Part print with two shaded views. Sizes in mm from the minimum x, y, z corner. A direction names the side the tool comes from. Round coordinates to 2 decimals unless told otherwise and drop trailing zeros. Write each loop counter-clockwise with the first axis right and the second up, starting at its lowest first coordinate (ties: lowest second). Pieces come first, ordered by that corner, then holes. Notation, with made-up numbers: M 51,2 L 58,2 A15 ccw 58,6 Z; hole C 48.25,78 d10. An arc over 180 degrees is marked long. One line per question, with ' | ' between items. Start each with the question number.
1) Mould opens along Y. For the marked faces 5, 6 and 7 say: pulls with the +Y half, pulls with the -Y half, needs draft (parallel to the pull), parting line crosses it, or undercut.
2) Wall check: probe 1 along Y at (x, z) = (84.5, 96.5); probe 2 along X at (y, z) = (21, 50); probe 3 along Z at (x, y) = (85, 14.75). Give the ranges that are in metal, low to high. Write a range as [from, to].
3) Tool access for the marked faces 1, 2, 3 and 4: list every direction of +Z, -Z, +X, -X, +Y, -Y with a clear straight run to the whole face (end or side of a thin tool).
4) Saw through at A-A (z = 80.5). List the corners of the cut face in (x, y).
5) Drop flat-ended pins along their axis: pin 1 Ø1.5 at (x, z) = (93.5, 89) entering from -Y; pin 2 Ø3 at (y, z) = (53, 62.5) entering from +X; pin 3 Ø22 at (y, z) = (22, 64) entering from -X. Give the stop position or say it passes through.
6) Saw through at B-B (x = 85). List the corners of the cut face in (y, z), plus the area to 3 significant figures.
7) Saw through at C-C (y = 56.5). List the corners of the cut face in (x, z).
8) Saw through at D-D (x = 63). List the corners of the cut face in (y, z), plus the area to 3 significant figures.
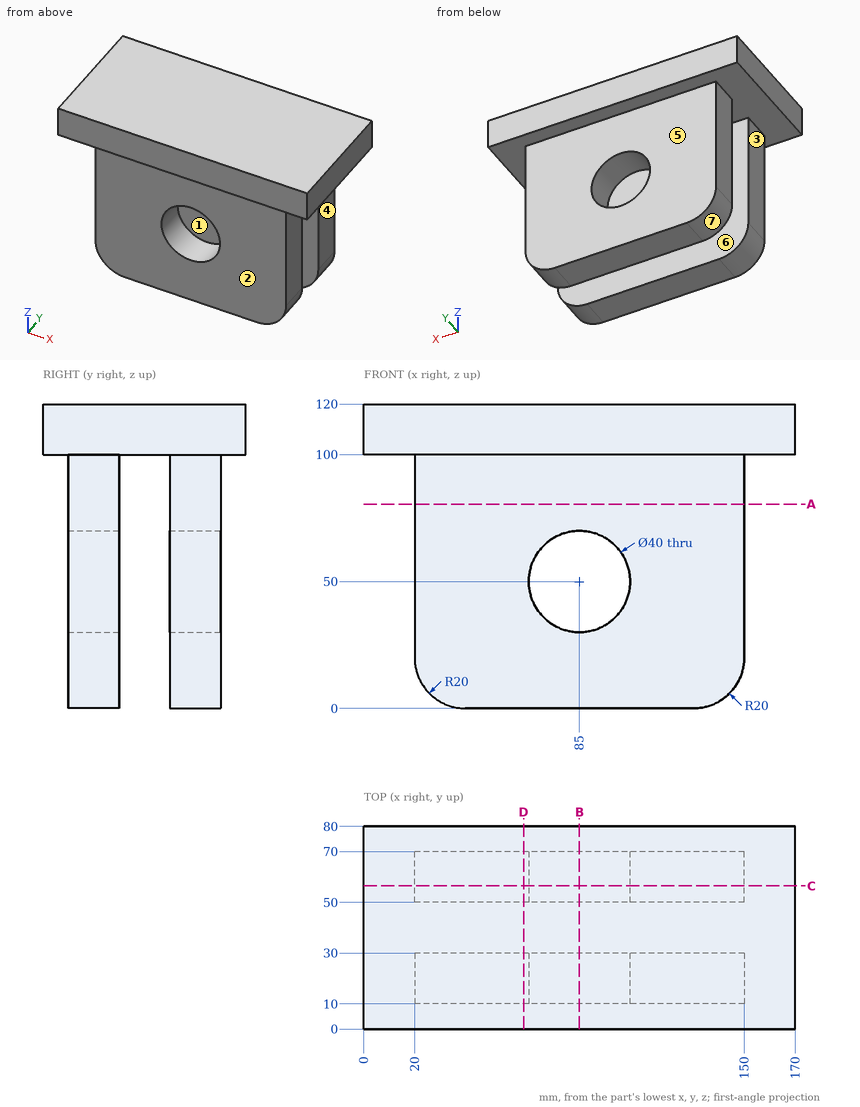
Answer key:
1) face 5: pulls with the +Y half | face 6: undercut | face 7: needs draft
2) probe 1: y = [10, 30], [50, 70] | probe 2: x = [20, 65], [105, 150] | probe 3: z = [0, 30], [70, 120]
3) face 1: -Z, +X, -X | face 2: -Z, +X, -X, -Y | face 3: -Z, -X, +Y, -Y | face 4: -Z, +X, +Y, -Y
4) outline: M 20,10 L 150,10 L 150,30 L 20,30 Z; M 20,50 L 150,50 L 150,70 L 20,70 Z
5) pin 1: stops at y = 10 | pin 2: stops at x = 150 | pin 3: stops at x = 20
6) outline: M 0,100 L 10,100 L 10,70 L 30,70 L 30,100 L 50,100 L 50,70 L 70,70 L 70,100 L 80,100 L 80,120 L 0,120 Z; M 10,0 L 30,0 L 30,30 L 10,30 Z; M 50,0 L 70,0 L 70,30 L 50,30 Z | area: 4,000 mm2
7) outline: M 0,100 L 20,100 L 20,20 A20 ccw 40,0 L 130,0 A20 ccw 150,20 L 150,100 L 170,100 L 170,120 L 0,120 Z; hole C 85,50 d40
8) outline: M 0,100 L 10,100 L 10,0 L 30,0 L 30,100 L 50,100 L 50,0 L 70,0 L 70,100 L 80,100 L 80,120 L 0,120 Z | area: 5,600 mm2
